Part model, mm, in its own coordinate system. Give positions to 0.01 mm unless a question says otherwise; leave off trailing zeros. Order: outer loops, then holes, each group sorted by start corner. A loop starts at its lowest first (then second) coordinate and runs counter-clockwise, first axis right, second up.
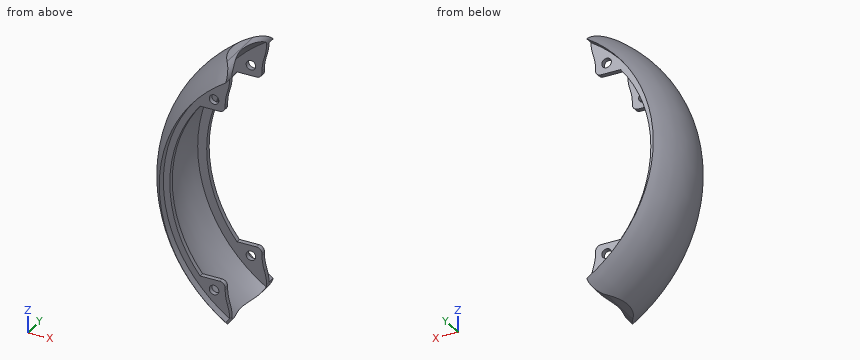
from build123d import *

# Parameters (mm, degrees)
REVOLVE1_ANGLE          = 120.922435
CUT_EXTRUDE1_DEPTH      = 120.118916294
CUT_EXTRUDE1_DEPTH_BACK = 120.118916294
BOSS_EXTRUDE2_DEPTH     = 2.5
CUT_EXTRUDE2_REACH      = 123.312
SKETCH5_R               = 2.6
MIRROR4_COPY_1_DEPTH    = 2.5
MIRROR4_COPY_2_REACH    = 123.312
MIRROR4_COPY_2_SKETCH_R = 2.6
FILLET2_R               = 25
FILLET3_START           = -21
FILLET3_DEPTH           = 42


with BuildPart() as part:
    # Revolve1: read off the stored shape, not the designer's step
    # Revolve1 outline → Revolve1 (revolve)
    with BuildSketch(Plane(origin=(0, 0, 0), x_dir=(-0.49301257198087967, 0, -0.8700221858486127), z_dir=(0.8700221858486127, 0, -0.49301257198087967))):
        with BuildLine():
            Line((78.5, 24), (78.5, 19.9))
            Line((78.5, 19.9), (75, 19.9))
            Line((75, 19.9), (75, 17.4))
            Line((75, 17.4), (79.88043342, 17.4))
            ThreePointArc((79.88043342, 17.4), (85.024521594, 0), (79.88043342, -17.4))
            Line((79.88043342, -17.4), (75, -17.4))
            Line((75, -17.4), (75, -19.9))
            Line((75, -19.9), (78.5, -19.9))
            Line((78.5, -19.9), (78.5, -24))
            ThreePointArc((78.5, -24), (88.024521594, 0), (78.5, 24))
        make_face()
    revolve(axis=Axis((0, 0, 0), (0, 1, 0)), revolution_arc=REVOLVE1_ANGLE)

    # Sketch3 → Cut-Extrude1 (cut, two sides: drawn at the far end of the back side and taken through both)
    with BuildSketch(Plane(origin=(0, 0, 0), x_dir=(1, 0, 0), z_dir=(0, 1, 0)).offset(-CUT_EXTRUDE1_DEPTH_BACK)):
        with BuildLine():
            Line((-42.5, -66), (-42.5, 66))
            ThreePointArc((-42.5, 66), (-43.964466094, 69.535533906), (-47.5, 71))
            Line((-47.5, 71), (-70.072780864, 71))
            Line((-70.072780864, 71), (-70.072780864, 87.352336772))
            Line((-70.072780864, 87.352336772), (-35.072780864, 87.352336772))
            Line((-35.072780864, 87.352336772), (-35.072780864, -87.352336772))
            Line((-35.072780864, -87.352336772), (-70.072780864, -87.352336772))
            Line((-70.072780864, -87.352336772), (-70.072780864, -71))
            Line((-70.072780864, -71), (-47.5, -71))
            ThreePointArc((-47.5, -71), (-43.964466094, -69.535533906), (-42.5, -66))
        make_face()
    extrude(amount=CUT_EXTRUDE1_DEPTH + CUT_EXTRUDE1_DEPTH_BACK, mode=Mode.SUBTRACT)

    # Sketch4 → Boss-Extrude2 (add)
    with BuildSketch(Plane.XZ.offset(-17.4)):
        with BuildLine():
            Line((-58.609991163, 46.796035472), (-48, 46.796035472))
            ThreePointArc((-48, 46.796035472), (-45.878679656, 47.674715128), (-45, 49.796035472))
            Line((-45, 49.796035472), (-45, 60))
            ThreePointArc((-45, 60), (-52.223976649, 53.829882621), (-58.609991163, 46.796035472))
        make_face()
    boss_extrude2 = extrude(amount=-BOSS_EXTRUDE2_DEPTH)

    # Sketch5 → Cut-Extrude2 (cut, up to next)
    with BuildSketch(Plane(origin=(0, 19.9, 0), x_dir=(1, 0, 0), z_dir=(0, 1, 0)), mode=Mode.PRIVATE) as cut_extrude2_sk1:
        with Locations(Location((-51, -52.496035472, 0), (0, 0, 270))):
            Circle(SKETCH5_R)
    cut_extrude2_tool1 = extrude(cut_extrude2_sk1.sketch, amount=-CUT_EXTRUDE2_REACH, mode=Mode.PRIVATE) & part.part
    cut_extrude2 = cut_extrude2_tool1.solids().sort_by_distance((-51, 19.9, 52.496035))[0]
    add(cut_extrude2, mode=Mode.SUBTRACT)

    # Mirror3: Boss-Extrude2, Cut-Extrude2 across plane
    add(boss_extrude2.mirror(Plane.XY))
    add(cut_extrude2.mirror(Plane.XY), mode=Mode.SUBTRACT)

    # Mirror4: Boss-Extrude2, Cut-Extrude2 across plane
    add(boss_extrude2.mirror(Plane.ZX))
    add(cut_extrude2.mirror(Plane.ZX), mode=Mode.SUBTRACT)

    # Mirror4 copy 1 sketch → Mirror4 copy 1 (add)
    with BuildSketch(Plane(origin=(0, -17.4, 0), x_dir=(1, 0, 0), z_dir=(0, 1, 0))):
        with BuildLine():
            Line((-58.609991163, 46.796035472), (-48, 46.796035472))
            ThreePointArc((-48, 46.796035472), (-45.878679656, 47.674715128), (-45, 49.796035472))
            Line((-45, 49.796035472), (-45, 60))
            ThreePointArc((-45, 60), (-52.223976649, 53.829882621), (-58.609991163, 46.796035472))
        make_face()
    extrude(amount=-MIRROR4_COPY_1_DEPTH)

    # Mirror4 copy 2 sketch → Mirror4 copy 2 (cut, up to next)
    with BuildSketch(Plane.XZ.offset(19.9), mode=Mode.PRIVATE) as mirror4_copy_2_sk1:
        with Locations(Location((-51, -52.496035472, 0), (0, 0, 270))):
            Circle(MIRROR4_COPY_2_SKETCH_R)
    mirror4_copy_2_tool1 = extrude(mirror4_copy_2_sk1.sketch, amount=-MIRROR4_COPY_2_REACH, mode=Mode.PRIVATE) & part.part
    add(mirror4_copy_2_tool1.solids().sort_by_distance((-51, -19.9, -52.496035))[0], mode=Mode.SUBTRACT)

    # Fillet2
    # the kernel refuses this fillet: 25 mm, written as the material it adds along each edge
    with BuildSketch(Plane(origin=(-45, 17.4, 60), x_dir=(0.8121446027945783, 0, 0.5834562058557923), z_dir=(0, 1, 0)), Plane(origin=(-45, -17.4, -60), x_dir=(0.812144602794579, 0, -0.5834562058557914), z_dir=(0, -1, 0))) as fillet2_piece_1:
        with BuildLine():
            CenterArc((14.993456513, 21.97790526), FILLET2_R, 215.694002743, 25.841932763)
            Line((-5.310158556, 7.391500113), (-5.716230858, 7.09977201))
            Line((-5.716230858, 7.09977201), (-0.406072301, -0.291728103))
            Line((-0.406072301, -0.291728103), (-0.010260898, -0.499894703))
            ThreePointArc((-0.010260898, -0.499894703), (1.539134774, -0.515794569), (2.83996581, -0.439558105))
            Line((2.83996581, -0.439558105), (3.078269549, 0))
        make_face()
    extrude(amount=2.5)
    with BuildSketch(Plane(origin=(-45, -17.4, 60), x_dir=(0.8121446027945783, 0, 0.5834562058557923), z_dir=(0, -1, 0)), Plane(origin=(-45, 17.4, -60), x_dir=(0.812144602794579, 0, -0.5834562058557914), z_dir=(0, 1, 0))) as fillet2_piece_2:
        with BuildLine():
            CenterArc((14.993456513, -21.97790526), FILLET2_R, 118.464064493, 25.841932763)
            Line((-5.310158556, -7.391500113), (-5.716230858, -7.09977201))
            Line((-5.716230858, -7.09977201), (-0.406072301, 0.291728103))
            Line((-0.406072301, 0.291728103), (-0.010260898, 0.499894703))
            ThreePointArc((-0.010260898, 0.499894703), (1.539134774, 0.515794569), (2.83996581, 0.439558105))
            Line((2.83996581, 0.439558105), (3.078269549, 0))
        make_face()
    extrude(amount=2.5)

    # Fillet3: read off the stored shape, not the designer's step
    # Fillet3 outline → Fillet3 (cut)
    with BuildSketch(Plane(origin=(0, 0, 0), x_dir=(1, 0, 0), z_dir=(0, 1, 0)).offset(FILLET3_START)):
        with BuildLine():
            ThreePointArc((-42.5, -61.796035472), (-43.174912338, -60.275537983), (-43.747209157, -58.713521457))
            ThreePointArc((-43.747209157, -58.713521457), (-42.852791856, -62.310406361), (-42.5, -66))
            Line((-42.5, -66), (-42.5, -61.796035472))
        make_face()
        with BuildLine():
            ThreePointArc((-42.5, 66), (-42.852791856, 62.310406361), (-43.747209157, 58.713521457))
            ThreePointArc((-43.747209157, 58.713521457), (-43.174912338, 60.275537983), (-42.5, 61.796035472))
            Line((-42.5, 61.796035472), (-42.5, 66))
        make_face()
    extrude(amount=FILLET3_DEPTH, mode=Mode.SUBTRACT)


solid = part.part
Item 1: Drop flat-ended pins along their axis: P1, Ø6, axis at y = 16.5, z = 37.5, coming from the -X side; P2, Ø0.8, axis at x = -55, y = 18, coming from the -Z side; P3, Ø3, axis at x = -56, y = -19, coming from the +Z side. Give the stop position or say it passes through.
Item 2: Band-saw the part on A-A on y = -11. List the corners of the cut face in (x, z).
Item 3: Drill centre lines: probe 1 along Z at (x, y) = (-50, -19); probe 2 along Z at (x, y) = (-65, -17.5); probe 3 along Y at (x, z) = (-80, -0.5). Where is each one in solid material? Low to high.
Working result:
1. P1: stops at x = -77.22
1. P2: stops at z = -62.69
1. P3: stops at z = 62.32
2. outline: (-48.97, -71) - (-47.5, -71) arc R5 ccw to (-44.61, -70.08) arc R83.07 cw to (-44.61, 70.08) arc R5 ccw to (-47.5, 71) - (-48.97, 71) arc R86.25 ccw to start
3. probe 1: z = -65.52 to -54.9, -50.1 to -46.8, 46.8 to 50.1, 54.9 to 65.52
3. probe 2: z = -52.15 to -37.42, 37.42 to 52.15
3. probe 3: y = -22.3 to -17.21, 17.21 to 22.3
